Autodesk Inventor part; units mm, degrees
ref_plane "YZ Plane" through (0, 0, 0) normal (1, 0, 0) x (0, 1, 0)
ref_plane "XZ Plane" through (0, 0, 0) normal (0, 1, 0) x (-1, 0, 0)
ref_plane "XY Plane" through (0, 0, 0) normal (0, 0, 1) x (1, 0, 0)
sketch "Sketch1" plane through (0, 0, 0) normal (0, 0, 1) x (1, 0, 0)
  line L0 (-212.471, -44.069) -> (212.471, -44.069)
  line L1 (212.471, -44.069) -> (212.471, 44.069)
  line L2 (212.471, 44.069) -> (-212.471, 44.069)
  line L3 (-212.471, 44.069) -> (-212.471, -44.069)
  line L4 (-212.471, -44.069) -> (212.471, 44.069) construction
  line L5 (212.471, -44.069) -> (-212.471, 44.069) construction
  point P0 (0, 0)
  dimension "d0" = 424.942
  dimension "d1" = 88.138
extrude "Extrusion1" add sketch "Sketch1" along normal blind 1.651
sketch "airflow" plane through (0, 0, 1.651) normal (0, 0, 1) x (1, 0, 0)
  line L0 (146.685, -25.019) -> (196.723, -25.019) construction
  line L1 (196.723, -25.019) -> (196.723, 25.019) construction
  line L2 (196.723, 25.019) -> (146.685, 25.019) construction
  line L3 (146.685, 25.019) -> (146.685, -25.019) construction
  line L4 (146.685, -25.019) -> (196.723, 25.019) construction
  line L5 (196.723, -25.019) -> (146.685, 25.019) construction
  line L6 (-212.471, 44.069) -> (-212.471, -44.069)
  line L7 (-212.471, -44.069) -> (212.471, -44.069)
  line L8 (-209.423, -35.814) -> (209.423, -35.814) construction
  line L9 (209.423, -35.814) -> (209.423, 35.814) construction
  line L10 (209.423, 35.814) -> (-209.423, 35.814) construction
  line L11 (-209.423, 35.814) -> (-209.423, -35.814) construction
  line L12 (-209.423, -35.814) -> (209.423, 35.814) construction
  line L13 (209.423, -35.814) -> (-209.423, 35.814) construction
  line L14 (150.622, -21.082) -> (192.786, -21.082)
  line L15 (192.786, -21.082) -> (192.786, 21.082)
  line L16 (192.786, 21.082) -> (150.622, 21.082)
  line L17 (150.622, 21.082) -> (150.622, -21.082)
  line L18 (150.622, -21.082) -> (192.786, 21.082) construction
  line L19 (192.786, -21.082) -> (150.622, 21.082) construction
  point P0 (0, 0)
  point P1 (171.704, 0)
  dimension "d4" = 50.038
  dimension "d5" = 50.038
  dimension "d10" = 44.069
  dimension "d11" = 8.255
  dimension "d12" = 3.048
  dimension "d13" = 12.7
  dimension "d14" = 3.937
hole "Hole1" at (196.723, 25.019, 1.651) at (146.685, 25.019, 1.651) at (196.723, -25.019, 1.651) at (146.685, -25.019, 1.651) direction (0, 0, -1) diameter 5.1054 end through all
extrude "Extrusion3" cut sketch "airflow" against normal through all
properties part number "NMT_backpanel"
Input: part model. Units: mm. Frame: model coordinates. Coordinates: 2 decimals unless noted, no trailing zeros. Loops run counter-clockwise (first coordinate to the right, second up) from the corner with the lowest first, then second, coordinate; pieces in that order, holes last.
(1) Section A-A on y = -16. Return the cut outline in (x, z), then the cut area to 3 significant figures.
(2) First-contact query: pin 1 Ø4 at (x, y) = (196.723, 25.019) entering from +Z. Flat tip, straight axial feed; report the tip coordinate or a pass-through.
(3) Section B-B on z = 0.35. Return the cut outline in (x, y) (3 decimals).
(4) Material intervals for probe 1 along X at (y, z) = (-25, 0.85); probe 2 along Y at (x, z) = (168, 0.75); probe 3 along X at (y, z) = (8, 1.3), sorted ascending.
Data:
1. outline: (-212.47, 0) - (150.62, 0) - (150.62, 1.65) - (-212.47, 1.65) - close; (192.79, 0) - (212.47, 0) - (212.47, 1.65) - (192.79, 1.65) - close
1. area: 632 mm2
2. pin 1: passes through
3. outline: (-212.471, -44.069) - (212.471, -44.069) - (212.471, 44.069) - (-212.471, 44.069) - close; hole circle Ø5.105 at (146.685, -25.019); hole circle Ø5.105 at (146.685, 25.019); hole (150.622, -21.082) - (192.786, -21.082) - (192.786, 21.082) - (150.622, 21.082) - close; hole circle Ø5.105 at (196.723, -25.019); hole circle Ø5.105 at (196.723, 25.019)
4. probe 1: x = -212.47 to 144.13, 149.24 to 194.17, 199.28 to 212.47
4. probe 2: y = -44.07 to -21.08, 21.08 to 44.07
4. probe 3: x = -212.47 to 150.62, 192.79 to 212.47
